Can you work these out from the model? Positions are in its coordinate system, mm. Face numbers are marked on the shaded views. A direction names the side the tool comes from. Give positions to 0.01 mm unless a question says otherwise; leave off trailing zeros. Order: outer loops, then holes, each group sorted by start corner. A loop starts at its lowest first (then second) coordinate and runs counter-clockwise, first axis right, second up.
Item 1: If I drill on line 1 along Y through (x, z) = (10.25, -1.3); line 2 along Z through (x, y) = (2.25, 1.7); line 3 along Z through (x, y) = (6.5, 0.35), over which ranges is the centre line in solid material (lowest first)?
Item 2: I want a section at B-B, the plane z = 1.6. Write out the boundary of the cut face in (x, y).
Item 3: I want a section at C-C, the plane x = 7.25. Write out the boundary of the cut face in (y, z), then the cut area to 3 significant figures.
Item 4: I'm going to push flat-ended pins straight in: pin 1 Ø3 at (x, z) = (7.5, -1.5) entering from +Y; pin 2 Ø3 at (y, z) = (0.5, -1) entering from -X. Where does each tip first touch, or does it pass through?
Item 5: I want a section at A-A, the plane y = 0. Write out the boundary of the cut face in (x, z).
Item 6: Which directions (+Z, -Z, +X, -X, +Y, -Y) give clear straight access to the entire face, cutting with the end or side of a thin tool? Please do the marked faces 1 and 2.
```python
from build123d import *

# Parameters (mm, degrees)
SKETCH1_R           = 2
BOSS_EXTRUDE1_DEPTH = 20.7
BOSS_EXTRUDE2_DEPTH = 2
CHAMFER1_SIZE       = 0.5


with BuildPart() as part:
    # Sketch1 → Boss-Extrude1 (new body)
    with BuildSketch(Plane(origin=(0, 0, 0), x_dir=(0, 0, -1), z_dir=(1, 0, 0))):
        Circle(SKETCH1_R)
    extrude(amount=BOSS_EXTRUDE1_DEPTH)

    # Sketch2 → Boss-Extrude2 (add)
    with BuildSketch(Plane(origin=(20.7, 0, 0), x_dir=(0, 0, -1), z_dir=(1, 0, 0))):
        Polygon((0, -2.886751346), (2.5, -1.443375673), (2.5, 1.443375673), (0, 2.886751346), (-2.5, 1.443375673), (-2.5, -1.443375673), align=None)
    extrude(amount=BOSS_EXTRUDE2_DEPTH)

    # Chamfer1
    chamfer1_edges = [part.edges().sort_by_distance(p)[0] for p in [
        (22.7, -2.165063509, 1.25),
        (22.7, -2.165063509, -1.25),
        (22.7, 0, -2.5),
        (22.7, 2.165063509, -1.25),
        (22.7, 2.165063509, 1.25),
        (22.7, 0, 2.5),
    ]]
    chamfer(chamfer1_edges, length=CHAMFER1_SIZE)


solid = part.part
```
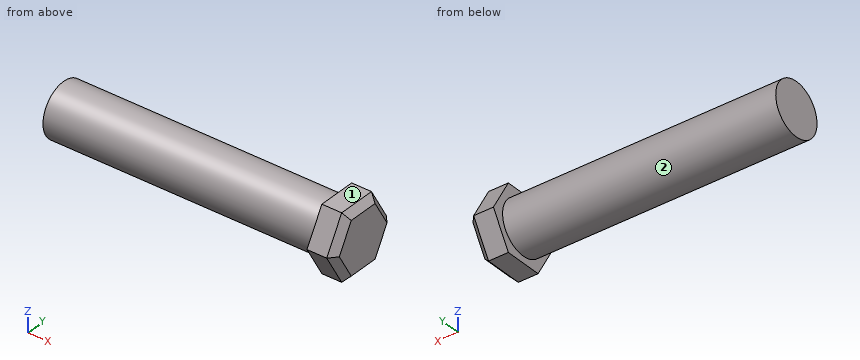
Results list:
1. line 1: y = -1.52 to 1.52
1. line 2: z = -1.05 to 1.05
1. line 3: z = -1.97 to 1.97
2. outline: (0, -1.2) - (20.7, -1.2) - (20.7, -1.96) - (22.2, -1.96) - (22.7, -1.39) - (22.7, 1.39) - (22.2, 1.96) - (20.7, 1.96) - (20.7, 1.2) - (0, 1.2) - close
3. outline: circle Ø4 at (0, 0)
3. area: 12.6 mm2
4. pin 1: stops at y = 2
4. pin 2: stops at x = 0
5. outline: (0, -2) - (20.7, -2) - (20.7, -2.5) - (22.2, -2.5) - (22.7, -2) - (22.7, 2) - (22.2, 2.5) - (20.7, 2.5) - (20.7, 2) - (0, 2) - close
6. face 1: +Z, +X, -X, +Y, -Y
6. face 2: -X
